```python
from build123d import *

# Parameters (mm, degrees)
F1_DEPTH = 4.25
F2_W     = 4
F2_H     = 12.7
F3_DEPTH = 1.5875
F4_R     = 1
F5_F1_R  = 0.4
F5_F2_R  = 0.4
F5_F3_R  = 0.4
F7_D     = 3


with BuildPart() as f1:
    # F0 (on Top) → F1 (new body)
    with BuildSketch(Plane.XY):
        Polygon((8.75, 106.9650896668), (-8.75, 106.9650896668), (-8.75, -147.0349103332), (2.75, -147.0349103332), (8.75, -127.0346005735), align=None)
    extrude(amount=-F1_DEPTH)

    # F2 (on face) → F3 (join)
    with BuildSketch(Plane.XY):
        Polygon((-2.75, 24.1850896668), (-8.75, 24.1850896668), (-8.75, 4.1850896668), align=None)
        Polygon((-2.75, -58.5949103332), (-8.75, -58.5949103332), (-8.75, -78.5949103332), align=None)
        with Locations((-6.75, -140.6849103332)):
            Rectangle(F2_W, F2_H)
        Polygon((-2.75, 106.9650896668), (-8.75, 106.9650896668), (-8.75, 86.9650896668), align=None)
    extrude(amount=F3_DEPTH)

    # F4
    f4_edges = [f1.edges().sort_by_distance(p)[0] for p in [
        (-2.75, -58.59491, 0.79375),
        (-8.75, -58.59491, 0.79375),
        (-2.75, 24.18509, 0.79375),
        (-8.75, 24.18509, 0.79375),
        (-2.75, 106.96509, 0.79375),
        (-8.75, 106.96509, -1.33125),
        (8.75, 106.96509, -2.125),
        (-8.75, -147.03491, -1.33125),
        (-4.75, -147.03491, 0.79375),
        (-4.75, -134.33491, 0.79375),
        (-8.75, -134.33491, 0.79375),
        (2.75, -147.03491, -2.125),
    ]]
    fillet(f4_edges, radius=F4_R)

    # F5: fillet of radius 0.4 on 3 edges, made by hand

    # F5_f1
    f5_f1_edges = [f1.edges().sort_by_distance(p)[0] for p in [
        (-8.75, 86.9650896668, 0.79375),
    ]]
    fillet(f5_f1_edges, radius=F5_F1_R)

    # F5_f2
    f5_f2_edges = [f1.edges().sort_by_distance(p)[0] for p in [
        (-8.75, -78.5949103332, 0.79375),
    ]]
    fillet(f5_f2_edges, radius=F5_F2_R)

    # F5_f3
    f5_f3_edges = [f1.edges().sort_by_distance(p)[0] for p in [
        (-8.75, 4.1850896668, 0.79375),
    ]]
    fillet(f5_f3_edges, radius=F5_F3_R)

    # F7 (through all)
    with Locations(Plane.XY):
        with Locations((1.113455, 100.5345896668), (1.113455, 81.1504351225), (1.113455, -18.4210048775), (1.113455, -37.9210048775), (1.113455, -108.6812892063), (1.113455, -128.0654437506)):
            Hole(F7_D / 2)


solid = f1.part
```
For this review, take the finished solid that the model builds, in its own axes (mm). A direction names the side the tool comes from. Round coordinates to 2 decimals unless told otherwise and drop trailing zeros. Write each loop counter-clockwise with the first axis right and the second up, starting at its lowest first coordinate (ties: lowest second). Pieces come first, ordered by that corner, then holes. Notation, with made-up numbers: (78.25, 26) - (88.25, 26) arc R5 cw to (88.25, 31) - close; hole circle Ø9 at (-21.5, 19.25). An arc over 180 degrees is marked (long way). Put each result on its own line as item: value.
Q1. Machinability: for faces 5 (the face through (-5.585, 97.514, 0.783)), 6 (the face through (-3, -147.035, -2)), which of the approach directions +Z, -Z, +X, -X, +Y, -Y give a long, thin tool a straight path to every point of the face, cutting with its end or side? Answer none if there is none.
Solved:
face 5: +Z, +X
face 6: +Z, -Z, +X, -X, -Y
Q2. We need section A-A (z = -0.9). Give the boundary of the cut face in (x, y), and give its area (3 significant figures).
Solved:
outline: (-8.75, -146.03) arc R1 ccw to (-7.75, -147.03) - (2.01, -147.03) arc R1 ccw to (2.96, -146.32) - (8.75, -127.03) - (8.75, 105.97) arc R1 ccw to (7.75, 106.97) - (-7.75, 106.97) arc R1 ccw to (-8.75, 105.97) - close; hole circle Ø3 at (1.11, -128.07); hole circle Ø3 at (1.11, -108.68); hole circle Ø3 at (1.11, -37.92); hole circle Ø3 at (1.11, -18.42); hole circle Ø3 at (1.11, 81.15); hole circle Ø3 at (1.11, 100.53)
area: 4,340 mm2
Q3. Mouldability with a two-part tool opening along Y and no side actions: class faces 1 (the face through (0, 106.965, -2)), 2 (the face through (5.816, -136.813, -2.095)), 3 (the face through (-7, 100, 1.588)), 4 (the face through (-2, -18, 0)) as released by +Y, released by -Y, zero draft, split by the parting line, or undercut.
Solved:
face 1: released by +Y
face 2: released by -Y
face 3: zero draft
face 4: undercut
Q4. We need section C-C (x = 5.5). Give the boundary of the cut face in (y, z), and give its area (3 significant figures).
Solved:
outline: (-137.87, -4.25) - (106.97, -4.25) - (106.97, 0) - (-137.87, 0) - close
area: 1,040 mm2
Q5. Insertion check: pin 1 Ø2.5 at (x, y) = (1.11, 81.15) entering from -Z; pin 2 Ø2 at (x, z) = (3.5, -2.5) entering from -Y; pin 3 Ø9 at (x, y) = (2, 1) entering from +Z; pin 4 Ø1.7 at (y, z) = (-138.5, 0.5) entering from +X. Each pin has a flat end and moves straight along its axis. Give the tip position at first contact, or say it passes through.
Solved:
pin 1: passes through
pin 2: stops at y = -146.9
pin 3: stops at z = 0
pin 4: stops at x = 5.52
Q6. Wall thickness on probe 1 along Z at (x, y) = (7, -21); probe 2 along X at (y, z) = (80.5, -3.25); probe 3 along X at (y, z) = (10, 0.4): over which ranges is each line inside the solid? List them lowest first.
Solved:
probe 1: z = -4.25 to 0
probe 2: x = -8.75 to -0.24, 2.47 to 8.75
probe 3: x = -8.75 to -7.01
Q7. We need section B-B (y = 59). Give the boundary of the cut face in (x, z).
Solved:
outline: (-8.75, -4.25) - (8.75, -4.25) - (8.75, 0) - (-8.75, 0) - close
